from build123d import *

# Parameters (mm, degrees)
BOSS_EXTRUDE1_DEPTH = 50
CUT_EXTRUDE1_START  = -8
CUT_EXTRUDE1_DEPTH  = 34
CUT_EXTRUDE2_DEPTH  = 34
SKETCH5_W           = 60
SKETCH5_H           = 65
BOSS_EXTRUDE3_DEPTH = 7


with BuildPart() as part:
    # Sketch2 → Boss-Extrude1 (new body)
    with BuildSketch(Plane(origin=(0, 0, 0), x_dir=(0, 0, -1), z_dir=(1, 0, 0))):
        with BuildLine():
            Line((40, 0), (0, 0))
            Line((0, 0), (10.700573851, 35))
            Line((10.700573851, 35), (15, 35))
            ThreePointArc((15, 35), (20, 30), (25, 35))
            Line((25, 35), (29.299426149, 35))
            Line((29.299426149, 35), (40, 0))
        make_face()
    extrude(amount=-BOSS_EXTRUDE1_DEPTH)

    # Sketch3 → Cut-Extrude1 (cut)
    with BuildSketch(Plane(origin=(0, 0, 0), x_dir=(0, 0, -1), z_dir=(1, 0, 0)).offset(CUT_EXTRUDE1_START)):
        Polygon((10.700573851, 35), (0, 0), (2.091383513, 0), (10.957573275, 29), (29.042426725, 29), (37.908616487, 0), (40, 0), (29.299426149, 35), (27.730888514, 35), (12.269111486, 35), align=None)
    extrude(amount=-CUT_EXTRUDE1_DEPTH, mode=Mode.SUBTRACT)

    # Sketch4 → Cut-Extrude2 (cut)
    with BuildSketch(Plane.XY):
        with BuildLine():
            Line((-11.388981029, 29), (-40.360215297, 29))
            ThreePointArc((-40.360215297, 29), (-25.874598163, 19.015151515), (-11.388981029, 29))
        make_face()
    extrude(amount=-CUT_EXTRUDE2_DEPTH, mode=Mode.SUBTRACT)

    # Sketch5 → Boss-Extrude3 (add)
    with BuildSketch(Plane.XZ):
        with Locations((-25, -20)):
            Rectangle(SKETCH5_W, SKETCH5_H)
    extrude(amount=BOSS_EXTRUDE3_DEPTH)


solid = part.part
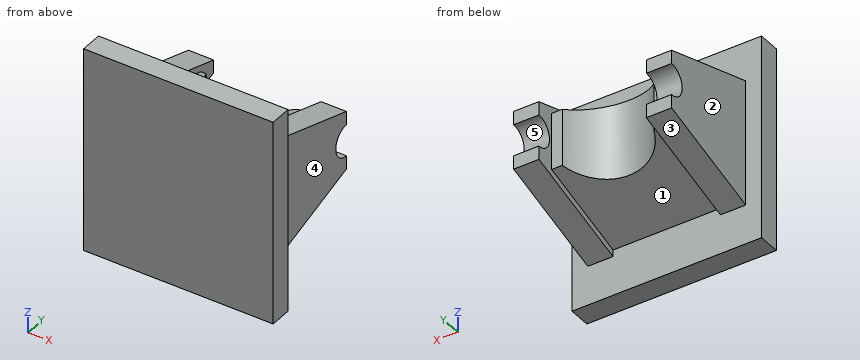
Build history of the part. All positions in model axes, mm. Face numbers are marked on the shaded views. A direction names the side the tool comes from. Round coordinates to 2 decimals unless told otherwise and drop trailing zeros. Write each loop counter-clockwise with the first axis right and the second up, starting at its lowest first coordinate (ties: lowest second). Pieces come first, ordered by that corner, then holes. Notation, with made-up numbers: (50.25, -29.75) - (81.25, -29.75) arc R17 ccw to (81.25, -21.75) - close; hole circle Ø2 at (-26.5, 37.25). An arc over 180 degrees is marked (long way). Use CSV: the item, a comma, the result in double quotes.
(1) Band-saw the part on C-C (y = 22.5). Write the cut outline in (x, z).
Response:
outline,"(-50, -33.12) - (-42, -33.12) - (-42, -31.03) - (-35.67, -31.03) - (-35.67, -8.97) - (-42, -8.97) - (-42, -6.88) - (-50, -6.88) - close; (-16.08, -31.03) - (-8, -31.03) - (-8, -33.12) - (0, -33.12) - (0, -6.88) - (-8, -6.88) - (-8, -8.97) - (-16.08, -8.97) - close"
(2) Pin check, flat tips, straight feed: P1, Ø0.8, axis at x = -41.5, z = -17, coming from the +Y side; P2, Ø12, axis at y = 22.5, z = -24.5, coming from the -X side; P3, Ø8, axis at x = -24, z = -33.5, coming from the +Y side. Stop position of each tip, or through.
Response:
P1,"y = 29"
P2,"x = -50"
P3,"y = 20.02"
(3) 3-axis set-ups, long thin cutter, end or side, ignore diameter. For the marked faces 4 and 5: which of +Z, -Z, +X, -X, +Y, -Y reach the whole face in a straight line?
Response:
face 4,"+Z, -Z, +X, +Y"
face 5,"+X, -X, +Y"
(4) Band-saw the part on D-D (y = 4). Write the cut outline in (x, z).
Response:
outline,"(-50, -38.78) - (-42, -38.78) - (-42, -36.69) - (-8, -36.69) - (-8, -38.78) - (0, -38.78) - (0, -1.22) - (-8, -1.22) - (-8, -3.31) - (-42, -3.31) - (-42, -1.22) - (-50, -1.22) - close"
(5) Band-saw the part on B-B (x = -1). Write the cut outline in (y, z), plus the area to 3 significant figures.
Response:
outline,"(-7, -52.5) - (0, -52.5) - (0, -40) - (35, -29.3) - (35, -25) arc R5 cw to (35, -15) - (35, -10.7) - (0, 0) - (0, 12.5) - (-7, 12.5) - close"
area,"1,440 mm²"
(6) Band-saw the part on A-A (z = -20). Write the cut outline in (x, y).
Response:
outline,"(-55, -7) - (5, -7) - (5, 0) - (0, 0) - (0, 30) - (-8, 30) - (-8, 29) - (-11.39, 29) arc R15.5 cw to (-40.36, 29) - (-42, 29) - (-42, 30) - (-50, 30) - (-50, 0) - (-55, 0) - close"
(7) Mould opens along X. For the marked faces 1, 2 and 3 say: pulls with the +X half, pulls with the -X half, needs draft (parallel to the pull), parting line crosses it, or undercut.
Response:
face 1,"undercut"
face 2,"pulls with the -X half"
face 3,"needs draft"
(8) Wall check: line 1 (X direction, y = 17.5, z = -33); line 2 (X direction, y = 16.5, z = -20.5); line 3 (Y direction, x = -21.5, z = 0). Give the ranges that are in metal, low to high.
Response:
line 1,"-50 to -42, -8 to 0"
line 2,"-50 to 0"
line 3,"-7 to 0"
